```python
from build123d import *

# Parameters (mm, degrees)
BOX003_W               = 14
BOX003_H               = 10
BOX003_DEPTH           = 10
BOX003_PLACEMENT_ANGLE = 45
BOX002_W               = 7
BOX002_H               = 1.6
BOX002_DEPTH           = 3
BOX001_W               = 7
BOX001_H               = 5
BOX001_DEPTH           = 1.7
BOX_W                  = 14
BOX_H                  = 7
BOX_DEPTH              = 10
CYLINDER_R             = 2.2
CYLINDER_DEPTH         = 13


with BuildPart() as obj1:
    # Box003 → Box003 (new body)
    with BuildSketch(Plane.XY):
        with Locations((7, 5)):
            Rectangle(BOX003_W, BOX003_H)
    extrude(amount=BOX003_DEPTH)


with BuildPart() as obj1_1:
    # Box003 placement: moved
    add(obj1.part.moved(Location((-4.7, -6.2, -3))).rotate(Axis((-4.7, -6.2, -3), (0, 0, 1)), BOX003_PLACEMENT_ANGLE))


with BuildPart() as obj2:
    # Box002 → Box002 (new body)
    with BuildSketch(Plane(origin=(1, -2.6, -1.5), x_dir=(1, 0, 0), z_dir=(0, 0, 1))):
        with Locations((3.5, 0.8)):
            Rectangle(BOX002_W, BOX002_H)
    extrude(amount=BOX002_DEPTH)


with BuildPart() as obj3:
    # Box001 → Box001 (new body)
    with BuildSketch(Plane(origin=(1, -4, -0.85), x_dir=(1, 0, 0), z_dir=(0, 0, 1))):
        with Locations((3.5, 2.5)):
            Rectangle(BOX001_W, BOX001_H)
    extrude(amount=BOX001_DEPTH)


with BuildPart() as obj4:
    # Box → Box (new body)
    with BuildSketch(Plane(origin=(-4, -0.5, -4), x_dir=(1, 0, 0), z_dir=(0, 0, 1))):
        with Locations((7, 3.5)):
            Rectangle(BOX_W, BOX_H)
    extrude(amount=BOX_DEPTH)


with BuildPart() as body:
    # Sketch → Revolution (revolve)
    with BuildSketch(Plane.XY):
        with BuildLine():
            add(Edge.make_bspline(
                [(1.699821, 2.2), (2.24, 1.1), (2.24, 0)],
                knots=[-2.2, -2.2, -2.2, 0, 0, 0], degree=2))
            Line((2.24, 0), (1.699821, 0))
            Line((1.699821, 0), (1.699821, 2.2))
        make_face()
    revolve(axis=Axis((0, 0, 0), (1, 0, 0)))


with BuildPart() as body_1:
    # Body placement: moved
    add(body.part.moved(Location((-1.7, 20, 0))))


with BuildPart() as cut004:
    # Cylinder → Cylinder (new body)
    with BuildSketch(Plane(origin=(-4, 0, 0), x_dir=(0, 0, -1), z_dir=(1, 0, 0))):
        Circle(CYLINDER_R)
    extrude(amount=CYLINDER_DEPTH)

    # Cut: cut Body
    add(body_1.part, mode=Mode.SUBTRACT)

    # Cut001: cut obj4
    add(obj4.part, mode=Mode.SUBTRACT)

    # Cut002: cut obj3
    add(obj3.part, mode=Mode.SUBTRACT)

    # Cut003: cut obj2
    add(obj2.part, mode=Mode.SUBTRACT)

    # Cut004: cut obj1
    add(obj1_1.part, mode=Mode.SUBTRACT)


solid = cut004.part
```
Could you check a few things on this model? Use its own coordinates, in mm. A direction names the side the tool comes from. Coordinates: 2 decimals unless noted, no trailing zeros. Order: outer loops, then holes, each group sorted by start corner. A loop starts at its lowest first (then second) coordinate and runs counter-clockwise, first axis right, second up. Notation, with made-up numbers: M 89.25,-28.75 L 100.25,-28.75 A19 ccw 100.25,-18.75 Z; hole C 26.5,86.5 d2. An arc over 180 degrees is marked long. Use one line per item in the form item = value. Start each with the question number.
1. Suppose I cut it at D-D on y = -1.5. Write out the boundary of the cut face in (x, z).
2. On a 3-axis mill with a long thin cutter (end or side, diameter ignored), from which of +Z, -Z, +X, -X, +Y, -Y can I reach the whole of each face in a straight line? I mean faces 4 (the flat face through (1, -1, 0)), 5 (the flat face through (9, -1, 0)). Say none if no direction works.
3. Please list where these lines run through material, in increasing order: line 1 (X direction, y = -1.45, z = -1.35); line 2 (X direction, y = -1.35, z = 0.1); line 3 (Z direction, x = 7.5, y = -1.2).
4. For pin 1 (0.7 mm diameter, centred on x = 4, y = -1.5, fed in from -Z); pin 2 (0.7 mm diameter, centred on x = 5.5, z = 1, fed in from -Y), each with a flat end and sliding along its axis, tell me the tip position at first contact or that it passes through.
5. Suppose I cut it at C-C on y = -1.9. Write out the boundary of the cut face in (x, z).
6. Suppose I cut it at B-B on z = -0.7. Write out the boundary of the cut face in (x, y).
7. Suppose I cut it at A-A on x = 1.75. Write out the boundary of the cut face in (y, z).
8. We'd pull the mould along X, two halves only. Please class faces 1 (the flat face through (5, -0.5, 1)), 2 (the flat face through (8, -1, 0)), 3 (the flat face through (0.3, -1.2, 0)): +X half, -X half, draft (parallel to the pull), parting line (faces both ways), or undercut.
Geometry says:
q1.outline = M 0,-1.61 L 9,-1.61 L 9,1.61 L 0,1.61 Z; hole M 1,-1.5 L 8,-1.5 L 8,1.5 L 1,1.5 Z
q2.face_4 = -Y
q2.face_5 = +Z, -Z, +X, +Y, -Y
q3.line_1 = 0.05 to 1, 8 to 9
q3.line_2 = 0.15 to 1, 8 to 9
q3.line_3 = -1.84 to -1.5, 1.5 to 1.84
q4.pin_1 = -1.88
q4.pin_2 = -1
q5.outline = M -0.4,-1.11 L 1,-1.11 L 1,1.11 L -0.4,1.11 Z; M 8,-1.11 L 9,-1.11 L 9,1.11 L 8,1.11 Z
q6.outline = M -0.59,-2.09 L 1,-2.09 L 1,-0.5 Z; M 8,-2.09 L 9,-2.09 L 9,-0.5 L 8,-0.5 Z
q7.outline = M -1.61,-1.5 A2.2 ccw -0.5,-2.14 L -0.5,-0.85 L -1,-0.85 L -1,-1.5 Z; M -1.61,1.5 L -1,1.5 L -1,0.85 L -0.5,0.85 L -0.5,2.14 A2.2 ccw Z
q8.face_1 = draft
q8.face_2 = undercut
q8.face_3 = -X half
